For this review, use the dimensioned drawing (mm, ordinates from the lowest corner) and the shaded views. Coordinates: 2 decimals unless noted, no trailing zeros. Loops run counter-clockwise (first coordinate to the right, second up) from the corner with the lowest first, then second, coordinate; pieces in that order, holes last. Notation, with made-up numbers: (-25.75, 7.25) - (13.25, 7.25) arc R21 ccw to (13.25, 14.25) - close; hole circle Ø10 at (4, -2). An arc over 180 degrees is marked (long way). Answer in a Markdown table with one row per item. Add a question column.
(1) We need section C-C, the plane z = 1.6. Write out the cut boundary in (x, y), plus the area to 3 significant figures.
(2) We need section A-A, the plane y = 80. Write out the cut boundary in (x, z), plus the area to 3 significant figures.
(3) Clearance check with flat-ended pins moving along their axes: pin 1 (1.5 mm diameter, centred on y = 70, z = 4, fed in from -X); pin 2 (12 mm diameter, centred on x = 40, y = 20.5, fed in from +Z); pin 3 (2.5 mm diameter, centred on x = 39, z = 1, fed in from +Y). State where each tip first meets the part, or that it passes through.
(4) We need section D-D, the plane y = 12.05. Write out the cut boundary in (x, z).
(5) To check wall thickness, follow L1, parallel to Y at x = 7.15, z = 2.95; L2, parallel to Y at x = 7.15, z = 4.1; L3, parallel to X at y = 6.9, z = 1.7. State the ranges of each line that lie inside material, in increasing order. Write a range as [from, to].
(6) We need section B-B, the plane x = 7.15. Write out the cut boundary in (y, z), plus the area to 4 significant figures.
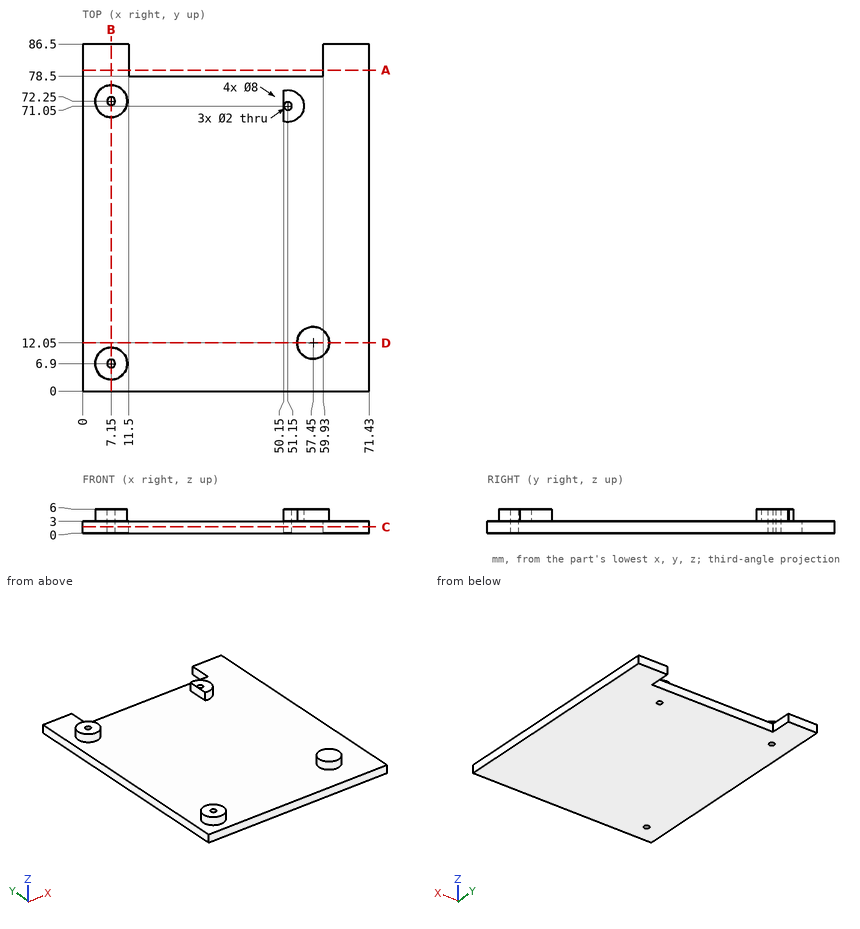
Responses:
| question | item | result |
|---|---|---|
| 1 | outline | (0, 0) - (71.43, 0) - (71.43, 86.5) - (59.93, 86.5) - (59.93, 78.5) - (11.5, 78.5) - (11.5, 86.5) - (0, 86.5) - close; hole circle Ø2 at (7.15, 6.9); hole circle Ø2 at (7.15, 72.25); hole circle Ø2 at (51.15, 71.05) |
| 1 | area | 5,780 mm2 |
| 2 | outline | (0, 0) - (11.5, 0) - (11.5, 3) - (0, 3) - close; (59.93, 0) - (71.43, 0) - (71.43, 3) - (59.93, 3) - close |
| 2 | area | 69.0 mm2 |
| 3 | pin 1 | stops at x = 3.44 |
| 3 | pin 2 | stops at z = 3 |
| 3 | pin 3 | stops at y = 78.5 |
| 4 | outline | (0, 0) - (71.43, 0) - (71.43, 3) - (61.45, 3) - (61.45, 6) - (53.45, 6) - (53.45, 3) - (0, 3) - close |
| 5 | L1 | y = [0, 5.9], [7.9, 71.25], [73.25, 86.5] |
| 5 | L2 | y = [2.9, 5.9], [7.9, 10.9], [68.25, 71.25], [73.25, 76.25] |
| 5 | L3 | x = [0, 6.15], [8.15, 71.43] |
| 6 | outline | (0, 0) - (5.9, 0) - (5.9, 6) - (2.9, 6) - (2.9, 3) - (0, 3) - close; (7.9, 0) - (71.25, 0) - (71.25, 6) - (68.25, 6) - (68.25, 3) - (10.9, 3) - (10.9, 6) - (7.9, 6) - close; (73.25, 0) - (86.5, 0) - (86.5, 3) - (76.25, 3) - (76.25, 6) - (73.25, 6) - close |
| 6 | area | 283.5 mm2 |
